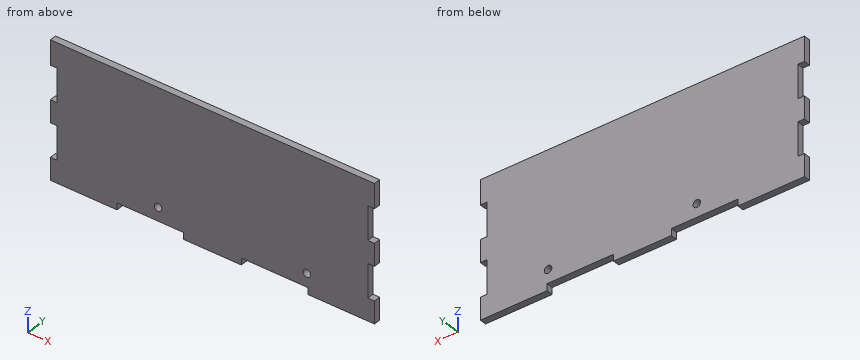
```python
from build123d import *

# Parameters (mm, degrees)
SKETCH1_W           = 146
SKETCH1_H           = 61
BOSS_EXTRUDE1_DEPTH = 3
SKETCH2_R           = 1.7
SKETCH2_W           = 3
SKETCH2_H           = 15
SKETCH2_W_2         = 30
SKETCH2_H_2         = 3
CUT_EXTRUDE1_DEPTH  = 10


with BuildPart() as part:
    # Sketch1 → Boss-Extrude1 (new body)
    with BuildSketch(Plane(origin=(0, 0, 0), x_dir=(1, 0, 0), z_dir=(0, 1, 0))):
        Rectangle(SKETCH1_W, SKETCH1_H)
    extrude(amount=BOSS_EXTRUDE1_DEPTH)

    # Sketch2 → Cut-Extrude1 (cut)
    with BuildSketch(Plane(origin=(0, 3, 0), x_dir=(1, 0, 0), z_dir=(0, 1, 0))):
        with Locations(Location((-24.5, 21.5, 0), (0, 0, 270))):
            Circle(SKETCH2_R)
        with Locations(Location((42.5, 21.5, 0), (0, 0, 270))):
            Circle(SKETCH2_R)
        with Locations((-71.5, 13)):
            Rectangle(SKETCH2_W, SKETCH2_H)
        with Locations((-71.5, -12)):
            Rectangle(SKETCH2_W, SKETCH2_H)
        with Locations((71.5, 13)):
            Rectangle(SKETCH2_W, SKETCH2_H)
        with Locations((71.5, -12)):
            Rectangle(SKETCH2_W, SKETCH2_H)
        with Locations((-28, 29)):
            Rectangle(SKETCH2_W_2, SKETCH2_H_2)
        with Locations((28, 29)):
            Rectangle(SKETCH2_W_2, SKETCH2_H_2)
    extrude(amount=-CUT_EXTRUDE1_DEPTH, mode=Mode.SUBTRACT)


solid = part.part
```
Could you check a few things on this model? Use its own coordinates, in mm. Give positions to 0.01 mm unless a question says otherwise; leave off trailing zeros. Write each loop counter-clockwise with the first axis right and the second up, starting at its lowest first coordinate (ties: lowest second). Pieces come first, ordered by that corner, then holes. Notation, with made-up numbers: (48.5, -8.75) - (101.5, -8.75) arc R30 ccw to (101.5, 15.25) - close; hole circle Ø5 at (-1, 67). An arc over 180 degrees is marked (long way). One line per item, written item: value. Start each with the question number.
Item 1: I'm going to push flat-ended pins straight in: pin 1 (1.5 mm diameter, centred on y = 2, z = 13, fed in from -X); pin 2 (0.9 mm diameter, centred on y = 1, z = 15.5, fed in from +X). Where does each tip first touch, or does it pass through?
Item 2: Please list where these lines run through material, in increasing order: line 1 (X direction, y = 0.7, z = -21.5); line 2 (Z direction, x = 37, y = 0.45); line 3 (X direction, y = 2.7, z = 5). Write a range as from..to.
Item 3: Imagine slicing it at A-A, the plane x = -24.5. List the corners of the cut face in (y, z) for me.
Item 4: Imagine slicing it at C-C, the plane z = 9. List the corners of the cut face in (x, y) for me, and give its area (3 significant figures).
Item 5: Imagine slicing it at B-B, the plane y = 0.9. Give the number of separate pieces and of enclosed holes in the cut face, and give its area (3 significant figures).
Item 6: Imagine slicing it at D-D, the plane x = 26. List the corners of the cut face in (y, z) for me, and give its area (3 significant figures).
Geometry says:
1. pin 1: x = -70
1. pin 2: x = 70
2. line 1: -73..-26.2, -22.8..40.8, 44.2..73
2. line 2: -27.5..30.5
2. line 3: -70..70
3. outline: (0, -27.5) - (3, -27.5) - (3, -23.2) - (0, -23.2) - close; (0, -19.8) - (3, -19.8) - (3, 30.5) - (0, 30.5) - close
4. outline: (-70, 0) - (70, 0) - (70, 3) - (-70, 3) - close
4. area: 420 mm^2
5. separate pieces: 1
5. enclosed holes: 2
5. area: 8,530 mm^2
6. outline: (0, -27.5) - (3, -27.5) - (3, 30.5) - (0, 30.5) - close
6. area: 174 mm^2
